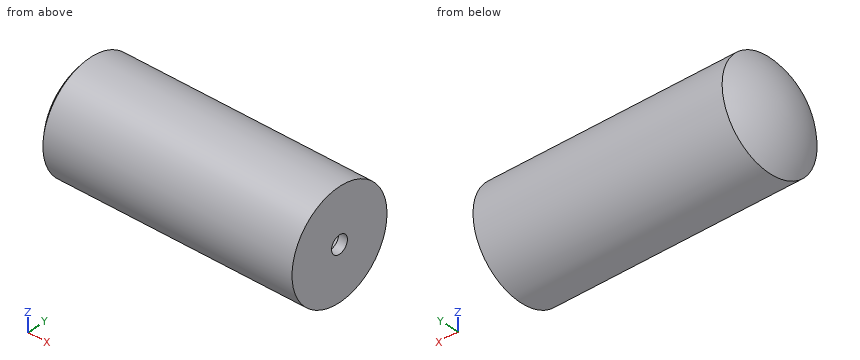
from build123d import *


with BuildPart() as part:
    # Sketch1 → Revolve6 (revolve)
    with BuildSketch(Plane.XY):
        with BuildLine():
            Line((169.943031877, 5), (169.943031877, 30))
            Line((169.943031877, 30), (29.943031877, 30))
            ThreePointArc((29.943031877, 30), (21.844861375, 15.961189352), (19.032566162, 0))
            Line((19.032566162, 0), (24.032566162, 0))
            ThreePointArc((24.032566162, 0), (26.168520101, 13.174839994), (32.357566788, 25))
            Line((32.357566788, 25), (164.943031877, 25))
            Line((164.943031877, 25), (164.943031877, 5))
            Line((164.943031877, 5), (169.943031877, 5))
        make_face()
    revolve(axis=Axis((0, 0, 0), (-1, 0, 0)))


solid = part.part
Model file for the job. Use its own axes, mm. Coordinates: 2 decimals unless noted, no trailing zeros. Loops run counter-clockwise (first coordinate to the right, second up) from the corner with the lowest first, then second, coordinate; pieces in that order, holes last. Notation, with made-up numbers: (31.25, 15.5) -> (58.25, 15.5) arc R28 cw to (58.25, 47.5) -> close; hole circle Ø8 at (-28.75, 47.5). An arc over 180 degrees is marked (long way). Use one line per item in the form item = value. Start each with the question number.
(1) Cut at D-D on z = 23. Give the cut face in (x, y), and give its area (3 significant figures).
(2) Cut at B-B on z = 0. Give the cut face in (x, y), and give its area (3 significant figures).
(3) Cut at A-A on y = 11. Give the cut face in (x, z), and give its area (3 significant figures).
(4) Probe probe 1 along Y at (x, z) = (85, 0); probe 2 along Z at (x, y) = (153, 1); probe 3 along Z at (x, y) = (168.9, 0). List the from-to ranges inside material, lowest first. Write a range as from..to.
(5) Flat gauge pins, fed straight in: pin 1 (4 mm diameter, centred on x = 100, z = -12, fed in from +Y); pin 2 (8 mm diameter, centred on y = -22, z = 1, fed in from -X); pin 3 (6 mm diameter, centred on x = 85.5, z = -16, fed in from +Y). Where does each tip first touch, or does it go through?
Values:
q1.outline = (29.94, -19.26) -> (169.94, -19.26) -> (169.94, 19.26) -> (29.94, 19.26) arc R40.64 ccw to start; hole (32.36, -9.8) -> (164.94, -9.8) -> (164.94, 9.8) -> (32.36, 9.8) arc R34.78 ccw to start
q1.area = 2,900 mm2
q2.outline = (29.94, -30) -> (169.94, -30) -> (169.94, -5) -> (164.94, -5) -> (164.94, -25) -> (32.36, -25) arc R41.7 cw to (32.36, 25) -> (164.94, 25) -> (164.94, 5) -> (169.94, 5) -> (169.94, 30) -> (29.94, 30) arc R46.7 ccw to start
q2.area = 1,880 mm2
q3.outline = (29.94, -27.91) -> (169.94, -27.91) -> (169.94, 27.91) -> (29.94, 27.91) arc R45.39 ccw to start; hole (32.36, -22.45) -> (164.94, -22.45) -> (164.94, 22.45) -> (32.36, 22.45) arc R40.22 ccw to start
q3.area = 2,020 mm2
q4.probe_1 = -30..-25, 25..30
q4.probe_2 = -29.98..-24.98, 24.98..29.98
q4.probe_3 = -30..-5, 5..30
q5.pin_1 = 28.28
q5.pin_2 = 22.65
q5.pin_3 = 27.04
